from build123d import *

# Parameters (mm, degrees)
SKETCH1_W           = 0.79375
SKETCH1_H           = 1.5875
SKETCH1_W_2         = 39.6875
SKETCH1_H_2         = 3.175
BOSS_EXTRUDE1_DEPTH = 9.525
SKETCH2_R           = 2.38125
CUT_EXTRUDE1_DEPTH  = 9.525


with BuildPart() as part:
    # Sketch1 → Boss-Extrude1 (new body)
    with BuildSketch(Plane.XY):
        with Locations((-19.446875, -2.38125)):
            Rectangle(SKETCH1_W, SKETCH1_H)
        with Locations((-17.065625, -2.38125)):
            Rectangle(SKETCH1_W, SKETCH1_H)
        with Locations((-14.684375, -2.38125)):
            Rectangle(SKETCH1_W, SKETCH1_H)
        with Locations((-12.303125, -2.38125)):
            Rectangle(SKETCH1_W, SKETCH1_H)
        with Locations((-9.921875, -2.38125)):
            Rectangle(SKETCH1_W, SKETCH1_H)
        with Locations((-7.540625, -2.38125)):
            Rectangle(SKETCH1_W, SKETCH1_H)
        with Locations((-5.159375, -2.38125)):
            Rectangle(SKETCH1_W, SKETCH1_H)
        with Locations((5.159375, -2.38125)):
            Rectangle(SKETCH1_W, SKETCH1_H)
        with Locations((7.540625, -2.38125)):
            Rectangle(SKETCH1_W, SKETCH1_H)
        with Locations((9.921875, -2.38125)):
            Rectangle(SKETCH1_W, SKETCH1_H)
        with Locations((12.303125, -2.38125)):
            Rectangle(SKETCH1_W, SKETCH1_H)
        with Locations((14.684375, -2.38125)):
            Rectangle(SKETCH1_W, SKETCH1_H)
        with Locations((17.065625, -2.38125)):
            Rectangle(SKETCH1_W, SKETCH1_H)
        with Locations((19.446875, -2.38125)):
            Rectangle(SKETCH1_W, SKETCH1_H)
        Rectangle(SKETCH1_W_2, SKETCH1_H_2)
    extrude(amount=BOSS_EXTRUDE1_DEPTH)

    # Sketch2 → Cut-Extrude1 (cut)
    with BuildSketch(Plane(origin=(0, 1.5875, 0), x_dir=(1, 0, 0), z_dir=(0, 1, 0))):
        with Locations(Location((0, -4.7625, 0), (0, 0, 270))):
            Circle(SKETCH2_R)
    extrude(amount=-CUT_EXTRUDE1_DEPTH, mode=Mode.SUBTRACT)


solid = part.part
Check sheet for the modelled part. Datum: model origin and axes. Units: mm. A direction names the side the tool comes from. Give positions to 0.01 mm unless a question says otherwise; leave off trailing zeros. Write each loop counter-clockwise with the first axis right and the second up, starting at its lowest first coordinate (ties: lowest second). Pieces come first, ordered by that corner, then holes. Notation, with made-up numbers: (60.5, 10.5) -> (119.5, 10.5) arc R15 ccw to (119.5, 27.5) -> close; hole circle Ø11 at (49.25, 23.5). An arc over 180 degrees is marked (long way). One line per item, written item: value. Start each with the question number.
Item 1: Section check C-C on y = -2.05. State how many separate pieces and enclosed holes the cut face has, then the cut area to 3 significant figures.
Item 2: Draft check along Z on faces 1 (the cylindrical face through (-1.449, 0.022, 2.873)), 2 (the flat face through (18, -1.588, 5)), 3 (the flat face through (0, 0, 0)). Enter one of: +Z half, -Z half, draft (parallel to the pull), parting line (faces both ways), or undercut.
Item 3: Tool access check on faces 4 (the flat face through (-16.669, -2, 5)), 5 (the flat face through (0, 1.588, 8)). Record the directions out of +Z, -Z, +X, -X, +Y, -Y that give a thin tool (end or side, any length) a straight path to the whole face; none if there is none.
Item 4: Section check A-A on x = 0. Record the cut outline in (y, z) (1 decimal).
Item 5: Section check D-D on x = -6. Record the cut outline in (y, z) (1 decimal), then the cut area to 3 significant figures.
Item 6: Section check B-B on y = 0.25. Record the cut outline in (x, z) (1 decimal), then the cut area to 3 significant figures.
Item 7: Material ranges on probe 1 along X at (y, z) = (-0.3, 4.75); probe 2 along Y at (x, z) = (18.5, 6.75); probe 3 along X at (y, z) = (1.45, 5.5), recorded low to high. Write a range as from..to.
Results list:
1. separate pieces: 14
1. enclosed holes: 0
1. area: 106 mm²
2. face 1: undercut
2. face 2: draft
2. face 3: -Z half
3. face 4: +Z, -Z, -Y
3. face 5: +Z, -Z, +X, -X, +Y
4. outline: (-1.6, 0) -> (1.6, 0) -> (1.6, 2.4) -> (-1.6, 2.4) -> close; (-1.6, 7.1) -> (1.6, 7.1) -> (1.6, 9.5) -> (-1.6, 9.5) -> close
5. outline: (-1.6, 0) -> (1.6, 0) -> (1.6, 9.5) -> (-1.6, 9.5) -> close
5. area: 30.2 mm²
6. outline: (-19.8, 0) -> (19.8, 0) -> (19.8, 9.5) -> (-19.8, 9.5) -> close; hole circle Ø4.8 at (0, 4.8)
6. area: 360 mm²
7. probe 1: -19.84..-2.38, 2.38..19.84
7. probe 2: -1.59..1.59
7. probe 3: -19.84..-2.26, 2.26..19.84
